from build123d import *

# Parameters (mm, degrees)
SKETCH1_R           = 9
SKETCH1_R_2         = 3
BOSS_EXTRUDE1_DEPTH = 3
BOSS_EXTRUDE5_DEPTH = 20
CHAMFER1_SIZE       = 2
CHAMFER2_SIZE       = 2
CHAMFER3_SIZE       = 2
CHAMFER4_SIZE       = 2
FILLET3_R           = 2
BOSS_EXTRUDE6_DEPTH = 35
CUT_EXTRUDE1_START  = -35
CUT_EXTRUDE1_DEPTH  = 35


with BuildPart() as part:
    # Sketch1 → Boss-Extrude1 (new body)
    with BuildSketch(Plane(origin=(0, 0, 0), x_dir=(1, 0, 0), z_dir=(0, 1, 0))):
        with BuildLine():
            Line((26.016071882, -39.591378024), (36.516071882, -39.591378024))
            ThreePointArc((36.516071882, -39.591378024), (40.051605788, -38.12691193), (41.516071882, -34.591378024))
            Line((41.516071882, -34.591378024), (41.516071882, -22.764050167))
            Line((41.516071882, -22.764050167), (41.516071882, 25.235949833))
            Line((41.516071882, 25.235949833), (55.516071882, 25.235949833))
            Line((55.516071882, 25.235949833), (55.516071882, 31.235949833))
            Line((55.516071882, 31.235949833), (67.773200773, 31.235949833))
            Line((67.773200773, 31.235949833), (67.773200773, 41.69443681))
            ThreePointArc((67.773200773, 41.69443681), (-56.98852563, 55.53324005), (-39.927712001, -68.828850188))
            Line((-39.927712001, -68.828850188), (-27.983928118, -68.828850188))
            Line((-27.983928118, -68.828850188), (-27.983928118, -48.591378024))
            Line((-27.983928118, -48.591378024), (-21.983928118, -48.591378024))
            Line((-21.983928118, -48.591378024), (-21.983928118, -39.591378024))
            Line((-21.983928118, -39.591378024), (26.016071882, -39.591378024))
        make_face()
        with Locations(Location((0, 0, 0), (0, 0, 270))):
            Circle(SKETCH1_R, mode=Mode.SUBTRACT)
        with Locations(Location((33, 0, 0), (0, 0, 270))):
            Circle(SKETCH1_R_2, mode=Mode.SUBTRACT)
        with Locations(Location((0, -33, 0), (0, 0, 270))):
            Circle(SKETCH1_R_2, mode=Mode.SUBTRACT)
        with Locations(Location((-33, 0, 0), (0, 0, 270))):
            Circle(SKETCH1_R_2, mode=Mode.SUBTRACT)
        with Locations(Location((0, 33, 0), (0, 0, 270))):
            Circle(SKETCH1_R_2, mode=Mode.SUBTRACT)
    extrude(amount=BOSS_EXTRUDE1_DEPTH)

    # Sketch2 → Boss-Extrude5 (add)
    with BuildSketch(Plane(origin=(0, 3, 0), x_dir=(1, 0, 0), z_dir=(0, 1, 0))):
        with BuildLine():
            Line((67.773200773, 39.156481082), (67.773200773, 44.853755219))
            ThreePointArc((67.773200773, 44.853755219), (62.937243445, 51.419543831), (57.467669607, 57.467669607))
            Line((57.467669607, 57.467669607), (55.346349264, 55.346349264))
            ThreePointArc((55.346349264, 55.346349264), (62.089724256, 47.658188126), (67.773200773, 39.156481082))
        make_face()
        with BuildLine():
            Line((-39.927712001, -76.985232291), (-39.927712001, -78.828850188))
            Line((-39.927712001, -78.828850188), (-36.927712001, -78.828850188))
            Line((-36.927712001, -78.828850188), (-36.927712001, -75.424551151))
            ThreePointArc((-36.927712001, -75.424551151), (-37.043512595, -73.56428019), (-37.389126407, -71.732731959))
            ThreePointArc((-37.389126407, -71.732731959), (-37.554188596, -71.15585041), (-37.753552772, -70.589907151))
            ThreePointArc((-37.753552772, -70.589907151), (-39.065927712, -68.356737552), (-41.023031213, -66.659940472))
            ThreePointArc((-41.023031213, -66.659940472), (-48.515602747, -61.422089217), (-55.346349264, -55.346349264))
            Line((-55.346349264, -55.346349264), (-57.467669607, -57.467669607))
            ThreePointArc((-57.467669607, -57.467669607), (-51.250804692, -63.074726465), (-44.490100887, -68.012476968))
            ThreePointArc((-44.490100887, -68.012476968), (-41.472337786, -71.100334086), (-40.037635444, -75.172604325))
            ThreePointArc((-40.037635444, -75.172604325), (-39.955218081, -76.077253312), (-39.927712001, -76.985232291))
        make_face()
        with BuildLine():
            Line((29.953228379, 72.313490189), (31.101278676, 75.085128787))
            ThreePointArc((31.101278676, 75.085128787), (0, 81.271557757), (-31.101278676, 75.085128787))
            Line((-31.101278676, 75.085128787), (-29.953228379, 72.313490189))
            ThreePointArc((-29.953228379, 72.313490189), (0, 78.271557757), (29.953228379, 72.313490189))
        make_face()
        with BuildLine():
            Line((-72.313490189, -29.953228379), (-75.085128787, -31.101278676))
            ThreePointArc((-75.085128787, -31.101278676), (-81.271557757, 0), (-75.085128787, 31.101278676))
            Line((-75.085128787, 31.101278676), (-72.313490189, 29.953228379))
            ThreePointArc((-72.313490189, 29.953228379), (-78.271557757, 0), (-72.313490189, -29.953228379))
        make_face()
    extrude(amount=BOSS_EXTRUDE5_DEPTH)

    # Chamfer1
    chamfer1_edges = [part.edges().sort_by_distance(p)[0] for p in [
        (67.773200773, 0, -36.465193321),
    ]]
    chamfer(chamfer1_edges, length=CHAMFER1_SIZE)

    # Chamfer2
    chamfer2_edges = [part.edges().sort_by_distance(p)[0] for p in [
        (55.516071882, 0, -28.235949833),
    ]]
    chamfer(chamfer2_edges, length=CHAMFER2_SIZE)

    # Chamfer3
    chamfer3_edges = [part.edges().sort_by_distance(p)[0] for p in [
        (-33.955820059, 0, 68.828850188),
    ]]
    chamfer(chamfer3_edges, length=CHAMFER3_SIZE)

    # Chamfer4
    chamfer4_edges = [part.edges().sort_by_distance(p)[0] for p in [
        (-24.983928118, 0, 48.591378024),
    ]]
    chamfer(chamfer4_edges, length=CHAMFER4_SIZE)

    # Fillet3
    fillet3_edges = [part.edges().sort_by_distance(p)[0] for p in [
        (67.773200773, 2.5, -41.69443681),
    ]]
    fillet(fillet3_edges, radius=FILLET3_R)

    # Sketch3 → Boss-Extrude6 (add)
    with BuildSketch(Plane(origin=(0, 23, 0), x_dir=(1, 0, 0), z_dir=(0, 1, 0))):
        with BuildLine():
            Line((67.773200773, 39.156481082), (67.773200773, 44.853755219))
            ThreePointArc((67.773200773, 44.853755219), (-57.621369969, 57.313557062), (-44.490100887, -68.012476968))
            ThreePointArc((-44.490100887, -68.012476968), (-41.472337786, -71.100334086), (-40.037635444, -75.172604325))
            ThreePointArc((-40.037635444, -75.172604325), (-39.955218081, -76.077253312), (-39.927712001, -76.985232291))
            Line((-39.927712001, -76.985232291), (-39.927712001, -78.828850188))
            Line((-39.927712001, -78.828850188), (-36.927712001, -78.828850188))
            Line((-36.927712001, -78.828850188), (-36.927712001, -75.424551151))
            ThreePointArc((-36.927712001, -75.424551151), (-37.043512595, -73.56428019), (-37.389126407, -71.732731959))
            ThreePointArc((-37.389126407, -71.732731959), (-37.554188596, -71.15585041), (-37.753552772, -70.589907151))
            ThreePointArc((-37.753552772, -70.589907151), (-39.065927712, -68.356737552), (-41.023031213, -66.659940472))
            ThreePointArc((-41.023031213, -66.659940472), (-54.572627392, 56.109402894), (67.773200773, 39.156481082))
        make_face()
    extrude(amount=BOSS_EXTRUDE6_DEPTH)

    # Sketch4 → Revolve1 (revolve)
    with BuildSketch(Plane(origin=(0, 0, 0), x_dir=(0, 0, -1), z_dir=(1, 0, 0)), mode=Mode.PRIVATE) as revolve1_sk:
        Polygon((79.448939848, 0), (81.178234321, 3), (79.448939848, 3), align=None)
    revolve(revolve1_sk.sketch.rotate(Axis((0, 0, 0), (0, -1, 0)), 207.35414034), axis=Axis((0, 0, 0), (0, -1, 0)))

    # Sketch5 → Cut-Extrude1 (cut)
    with BuildSketch(Plane(origin=(0, 3, 0), x_dir=(1, 0, 0), z_dir=(0, 1, 0)).offset(CUT_EXTRUDE1_START)):
        with BuildLine():
            Line((67.773200773, 44.684437834), (67.773200773, 41.459948143))
            ThreePointArc((67.773200773, 41.459948143), (57.505508315, -54.8201656), (-38.173959697, -69.676989344))
            ThreePointArc((-38.173959697, -69.676989344), (-37.949405437, -70.126839575), (-37.753552772, -70.589907151))
            ThreePointArc((-37.753552772, -70.589907151), (-37.554188596, -71.15585041), (-37.389126407, -71.732731959))
            ThreePointArc((-37.389126407, -71.732731959), (-37.343653711, -71.916668059), (-37.300507998, -72.101163864))
            ThreePointArc((-37.300507998, -72.101163864), (60.347870238, -54.295858822), (67.773200773, 44.684437834))
        make_face()
    extrude(amount=CUT_EXTRUDE1_DEPTH, mode=Mode.SUBTRACT)


solid = part.part
Read the model definition and answer for the solid it produces. Units are mm, in the model's axes. A direction names the side the tool comes from. Give positions to 0.01 mm unless a question says otherwise; leave off trailing zeros. Write each loop counter-clockwise with the first axis right and the second up, starting at its lowest first coordinate (ties: lowest second). Pieces come first, ordered by that corner, then holes. Notation, with made-up numbers: M 57,54.5 L 105,54.5 A24 cw 105,83.5 Z; hole C -12,85.5 d2. An arc over 180 degrees is marked long. One line per item, written item: value. Start each with the question number.
(1) Find section A-A (z = 0). Determine the outline of the cut face in (x, y).
(2) Find the intervals of material crossed by line 1 (X direction, y = 2.2, z = 0); line 2 (X direction, y = 1, z = 0); line 3 (X direction, y = 44, z = 0), in increasing order.
(3) Find section D-D (x = -33). Give the number of separate pieces and of enclosed holes in the cut face, plus the area to 3 significant figures.
(4) Determine the mould class of faces 3 (the cylindrical face through (-41.505, 30.115, 71.049)), 4 (the cylindrical face through (-35.662, 1.479, 1.384)), 5 (the flat face through (-66, 23, 44)) for opening direction Z: pulls with the +Z half, pulls with the -Z half, needs draft (parallel to the pull), parting line crosses it, or undercut.
(5) Find section B-B (x = 0). Determine the outline of the cut face in (y, z).
(6) Find section C-C (y = 36). Determine the outline of the cut face in (x, z), plus the area to 3 significant figures.
(7) A tool of negligible diameter and unlimited length cuts with its end or side. For faces 1 (the flat face through (-40, 3, 74)), 2 (the cylindrical face through (0, 1, 30)), from which of +Z, -Z, +X, -X, +Y, -Y can it reach the whole face along a straight path? Write none if from no direction.
(8) Flat-ended cylindrical pins translate along their axes: pin 1 Ø2.5 at (y, z) = (39.5, 78) entering from +X; pin 2 Ø8 at (x, y) = (44, 22.5) entering from +Z; pin 3 Ø3.5 at (x, y) = (45.5, 2) entering from +Z. Find the tip coordinate at first contact, or state that the pin passes through.
Results below:
1. outline: M -81.27,3 L -81.18,3 L -79.57,0.21 L -79.57,0 L -36,0 L -36,3 L -78.27,3 L -78.27,58 L -81.27,58 Z; M -30,0 L -9,0 L -9,3 L -30,3 Z; M 9,0 L 30,0 L 30,3 L 9,3 Z; M 36,0 L 41.52,0 L 41.52,3 L 36,3 Z
2. line 1: x = -80.72 to -36, -30 to -9, 9 to 30, 36 to 41.52
2. line 2: x = -80.03 to -36, -30 to -9, 9 to 30, 36 to 41.52
2. line 3: x = -81.27 to -78.27
3. separate pieces: 3
3. enclosed holes: 0
3. area: 521 mm^2
4. face 3: pulls with the +Z half
4. face 4: undercut
4. face 5: needs draft
5. outline: M 0,-79.57 L 0.21,-79.57 L 3,-81.18 L 3,-81.27 L 58,-81.27 L 58,-78.27 L 3,-78.27 L 3,-36 L 0,-36 Z; M 0,-30 L 3,-30 L 3,-9 L 0,-9 Z; M 0,9 L 3,9 L 3,30 L 0,30 Z; M 0,36 L 3,36 L 3,39.59 L 0,39.59 Z
6. outline: M -44.49,68.01 A81.27 ccw long 67.77,-44.85 L 67.77,-39.16 A78.27 cw long -41.02,66.66 A8 ccw -37.75,70.59 A10 ccw -37.39,71.73 A15 ccw -36.93,75.42 L -36.93,78.83 L -39.93,78.83 L -39.93,76.99 A15 cw -40.04,75.17 A10 cw Z
6. area: 902 mm^2
7. face 1: +Z, -X, -Y
7. face 2: +Y, -Y
8. pin 1: stops at x = -36.93
8. pin 2: stops at z = -61.85
8. pin 3: stops at z = -25.24
